Work out the finished part from the listing and answer in its coordinate system (mm). A direction names the side the tool comes from. Give positions to 0.01 mm unless a question says otherwise; leave off trailing zeros. Order: outer loops, then holes, each group sorted by start corner. A loop starts at its lowest first (then second) coordinate and runs counter-clockwise, first axis right, second up.
```python
from build123d import *

# Parameters (mm, degrees)
BOSS_EXTRUDE1_DEPTH = 6
SKETCH2_R           = 8.125
CUT_EXTRUDE1_DEPTH  = 5
SKETCH3_R           = 1.5
CUT_EXTRUDE2_DEPTH  = 0.5
SKETCH4_R           = 1.65
CUT_EXTRUDE3_DEPTH  = 21
SKETCH5_W           = 20
SKETCH5_H           = 0.05
CUT_EXTRUDE4_DEPTH  = 7
FILLET1_R           = 1
CHAMFER1_SIZE       = 0.5


with BuildPart() as part:
    # Sketch1 → Boss-Extrude1 (new body)
    with BuildSketch(Plane.XY):
        Polygon((-3.170042294, -13.5), (10, -13.5), (10, 13.5), (10, 16.5), (-10, 16.5), (-10, 13.5), (-10, -13), (-3.670042294, -13), align=None)
    extrude(amount=BOSS_EXTRUDE1_DEPTH)

    # Sketch2 → Cut-Extrude1 (cut)
    with BuildSketch(Plane.XY.offset(6)):
        Circle(SKETCH2_R)
    extrude(amount=-CUT_EXTRUDE1_DEPTH, mode=Mode.SUBTRACT)

    # Sketch3 → Cut-Extrude2 (cut)
    with BuildSketch(Plane(origin=(10, 0, 0), x_dir=(0, 0, -1), z_dir=(1, 0, 0))):
        with Locations((-3, 0)):
            Circle(SKETCH3_R)
    extrude(amount=-CUT_EXTRUDE2_DEPTH, mode=Mode.SUBTRACT)

    # Sketch4 → Cut-Extrude3 (cut, through all)
    with BuildSketch(Plane(origin=(10, 0, 0), x_dir=(0, 0, -1), z_dir=(1, 0, 0))):
        with Locations((-3, 13.32)):
            Circle(SKETCH4_R)
        with Locations((-3, -10.31539104)):
            Circle(SKETCH4_R)
    extrude(amount=-CUT_EXTRUDE3_DEPTH, mode=Mode.SUBTRACT)

    # Sketch5 → Cut-Extrude4 (cut, through all)
    with BuildSketch(Plane(origin=(0, 0, 0), x_dir=(-1, 0, 0), z_dir=(0, 0, -1))):
        with Locations((0, 16.475)):
            Rectangle(SKETCH5_W, SKETCH5_H)
        with Locations((0, -13.475)):
            Rectangle(SKETCH5_W, SKETCH5_H)
    extrude(amount=-CUT_EXTRUDE4_DEPTH, mode=Mode.SUBTRACT)

    # Fillet1
    fillet1_edges = [part.edges().sort_by_distance(p)[0] for p in [
        (-10, -13, 3),
        (-10, 16.45, 3),
        (10, 16.45, 3),
        (-3.220042294, -13.45, 3),
        (10, -13.45, 3),
    ]]
    fillet(fillet1_edges, radius=FILLET1_R)

    # Chamfer1
    chamfer1_edges = [part.edges().sort_by_distance(p)[0] for p in [
        (-9.707106781, 16.157106781, 0),
        (9.707106781, -13.157106781, 0),
        (-3.188512164, -13.373879533, 0),
        (-3.591488904, -13.078553391, 6),
        (-8.125, 0, 6),
        (0, 16.45, 6),
        (-10, 1.725, 6),
        (-6.335021147, -13, 6),
        (3.097085634, -13.45, 6),
        (10, 1.5, 6),
        (-9.707106781, -12.707106781, 6),
        (9.707106781, 16.157106781, 6),
        (-9.707106781, 16.157106781, 6),
        (9.707106781, -13.157106781, 6),
        (-3.591488904, -13.078553391, 0),
        (-3.188512164, -13.373879533, 6),
        (3.097085634, -13.45, 0),
        (-10, 1.725, 0),
        (0, 16.45, 0),
        (10, 1.5, 0),
        (-6.335021147, -13, 0),
        (-9.707106781, -12.707106781, 0),
        (9.707106781, 16.157106781, 0),
    ]]
    chamfer(chamfer1_edges, length=CHAMFER1_SIZE)


solid = part.part
```
1. The mould has two halves that part along X. Classify faces 1 (the face through (7.75, 2.44, 3.28)), 2 (the face through (9.5, 0, 3)), 3 (the face through (-9.715, 16.149, 3.035)): pulls with the +X half, pulls with the -X half, needs draft (parallel to the pull), parting line crosses it, or undercut.
Findings below:
face 1: undercut
face 2: pulls with the +X half
face 3: pulls with the -X half
2. The part is cut by section C-C (x = 0). Write down the section's boundary in (y, z) (3 decimals), then the cut area to 3 significant figures.
Findings below:
outline: (-13.45, 0.5) - (-12.95, 0) - (15.95, 0) - (16.45, 0.5) - (16.45, 5.5) - (15.95, 6) - (8.625, 6) - (8.125, 5.5) - (8.125, 1) - (-8.125, 1) - (-8.125, 5.5) - (-8.625, 6) - (-12.95, 6) - (-13.45, 5.5) - close; hole circle Ø3.3 at (-10.315, 3); hole circle Ø3.3 at (13.32, 3)
area: 80.3 mm2
3. The part is cut by section B-B (z = 3). Write down the section's boundary in (x, y) (3 decimals), then the cut area to 3 significant figures.
Findings below:
outline: (-10, -12) arc R1 ccw to (-9, -13) - (-3.67, -13) - (-3.513, -13.157) arc R1 ccw to (-2.806, -13.45) - (9, -13.45) arc R1 ccw to (10, -12.45) - (10, -11.965) - (-10, -11.965) - close; (-10, -8.665) - (10, -8.665) - (10, -1.5) - (9.5, -1.5) - (9.5, 1.5) - (10, 1.5) - (10, 11.67) - (-10, 11.67) - close; (-10, 14.97) - (10, 14.97) - (10, 15.45) arc R1 ccw to (9, 16.45) - (-9, 16.45) arc R1 ccw to (-10, 15.45) - close; hole circle Ø16.25 at (0, 0)
area: 253 mm2
4. Given P1, Ø2.5, axis at y = 0, z = 3, coming from the +X side; P2, Ø2, axis at x = -1, y = -1, coming from the +Z side; P3, Ø8, axis at x = -2.5, y = -3.5, coming from the +Z side, each flat-ended and moving along its own axis, determine where each tip first touches the part or whether it passes through.
Findings below:
P1: stops at x = 9.5
P2: stops at z = 1
P3: stops at z = 5.68
5. The part is cut by section A-A (y = 13.32). Write down the section's boundary in (x, z), then the cut area to 3 significant figures.
Findings below:
outline: (-10, 0.5) - (-9.5, 0) - (9.5, 0) - (10, 0.5) - (10, 1.35) - (-10, 1.35) - close; (-10, 4.65) - (10, 4.65) - (10, 5.5) - (9.5, 6) - (-9.5, 6) - (-10, 5.5) - close
area: 53.5 mm2
6. Which of the six approach directions +Z, -Z, +X, -X, +Y, -Y give full straight-line access (tool end or side, diameter ignored) to faces 4 (the face through (-6, -13, 3)), 5 (the face through (0, 0, 1)), 6 (the face through (9.75, 0.45, 1.57))?
Findings below:
face 4: +Z, -Z, -X, -Y
face 5: +Z
face 6: +X
7. Straight lines are drawn through the part: probe 1 along Y at (x, z) = (0, 3.9) (3 decimals); probe 2 along Y at (x, z) = (1.25, 3); probe 3 along Z at (x, y) = (5.25, 3.5). For each, find the intervals that lie inside material, in ascending order.
Findings below:
probe 1: y = -13.45 to -11.698, -8.932 to -8.125, 8.125 to 11.937, 14.703 to 16.45
probe 2: y = -13.45 to -11.97, -8.67 to -8.03, 8.03 to 11.67, 14.97 to 16.45
probe 3: z = 0 to 1
8. The part is cut by section D-D (y = 0). Write down the section's boundary in (x, z) (3 decimals), then the cut area to 3 significant figures.
Findings below:
outline: (-10, 0.5) - (-9.5, 0) - (9.5, 0) - (10, 0.5) - (10, 1.5) - (9.5, 1.5) - (9.5, 4.5) - (10, 4.5) - (10, 5.5) - (9.5, 6) - (8.625, 6) - (8.125, 5.5) - (8.125, 1) - (-8.125, 1) - (-8.125, 5.5) - (-8.625, 6) - (-9.5, 6) - (-10, 5.5) - close
area: 36.5 mm2
